```python
from build123d import *

# Parameters (mm, degrees)
SKETCH1_W           = 6.8
SKETCH1_H           = 5
BOSS_EXTRUDE1_DEPTH = 3.8
SKETCH3_W           = 2.8
SKETCH3_H           = 2.9
CUT_EXTRUDE2_DEPTH  = 10.340235543
SKETCH4_W           = 1.9
SKETCH4_H           = 0.2
CUT_EXTRUDE3_DEPTH  = 2.2
HOLE1_D             = 1.05
HOLE1_CBORE_D       = 1.3
HOLE1_CBORE_DEPTH   = 1.2
CUT_EXTRUDE8_DEPTH  = 10.340235543
CUT_EXTRUDE9_DEPTH  = 10.340235543
CUT_EXTRUDE10_DEPTH = 0.3
SKETCH20_W          = 5
SKETCH20_H          = 1.3
CUT_EXTRUDE11_DEPTH = 0.3


with BuildPart() as part:
    # Sketch1 → Boss-Extrude1 (new body)
    with BuildSketch(Plane(origin=(0, 4, 0), x_dir=(-1, 0, 0), z_dir=(0, 1, 0))):
        with Locations((-3.4, 2.5)):
            Rectangle(SKETCH1_W, SKETCH1_H)
    extrude(amount=-BOSS_EXTRUDE1_DEPTH)

    # Sketch3 → Cut-Extrude2 (cut, through all)
    with BuildSketch(Plane.XY.offset(5)):
        with Locations((3.2, 1.65)):
            Rectangle(SKETCH3_W, SKETCH3_H)
    extrude(amount=-CUT_EXTRUDE2_DEPTH, mode=Mode.SUBTRACT)

    # Sketch4 → Cut-Extrude3 (cut)
    with BuildSketch(Plane(origin=(6.8, 0, 0), x_dir=(0, 0, -1), z_dir=(1, 0, 0))):
        with Locations((-1.9, 0.3)):
            Rectangle(SKETCH4_W, SKETCH4_H)
    extrude(amount=-CUT_EXTRUDE3_DEPTH, mode=Mode.SUBTRACT)

    # Hole1 (through all)
    with Locations(Plane(origin=(0, 0, 0), x_dir=(-1, 0, 0), z_dir=(0, 0, -1))):
        with Locations((-5.7, 1.7), (-0.7, 1.7)):
            CounterBoreHole(HOLE1_D / 2, HOLE1_CBORE_D / 2, HOLE1_CBORE_DEPTH)

    # Sketch17 → Cut-Extrude8 (cut, through all)
    with BuildSketch(Plane.XY.offset(5)):
        with BuildLine():
            Line((6.8, 2.225), (5.7, 2.225))
            ThreePointArc((5.7, 2.225), (6.07123106, 2.07123106), (6.225, 1.7))
            ThreePointArc((6.225, 1.7), (6.07123106, 1.32876894), (5.7, 1.175))
            Line((5.7, 1.175), (6.8, 1.175))
            Line((6.8, 1.175), (6.8, 2.225))
        make_face()
        with BuildLine():
            ThreePointArc((6.225, 1.7), (6.07123106, 2.07123106), (5.7, 2.225))
            Line((5.7, 2.225), (5.7, 1.175))
            ThreePointArc((5.7, 1.175), (6.07123106, 1.32876894), (6.225, 1.7))
        make_face()
        with BuildLine():
            Line((5.7, 1.175), (5.7, 2.225))
            ThreePointArc((5.7, 2.225), (5.175, 1.7), (5.7, 1.175))
        make_face()
    extrude(amount=-CUT_EXTRUDE8_DEPTH, mode=Mode.SUBTRACT)

    # Sketch18 → Cut-Extrude9 (cut, through all)
    with BuildSketch(Plane(origin=(6.8, 0, 0), x_dir=(0, 0, -1), z_dir=(1, 0, 0))):
        Polygon((-1.288675135, 4), (-3.711324865, 4), (-4, 3.5), (-1, 3.5), align=None)
    extrude(amount=-CUT_EXTRUDE9_DEPTH, mode=Mode.SUBTRACT)

    # Sketch19 → Cut-Extrude10 (cut)
    with BuildSketch(Plane(origin=(0, 3.5, 0), x_dir=(1, 0, 0), z_dir=(0, 1, 0))):
        with BuildLine():
            Line((6.8, -1.75), (6, -1.75))
            ThreePointArc((6, -1.75), (6.530330086, -1.969669914), (6.75, -2.5))
            ThreePointArc((6.75, -2.5), (6.530330086, -3.030330086), (6, -3.25))
            Line((6, -3.25), (6.8, -3.25))
            Line((6.8, -3.25), (6.8, -1.75))
        make_face()
        with BuildLine():
            ThreePointArc((6.75, -2.5), (6.530330086, -1.969669914), (6, -1.75))
            Line((6, -1.75), (6, -3.25))
            ThreePointArc((6, -3.25), (6.530330086, -3.030330086), (6.75, -2.5))
        make_face()
        with BuildLine():
            Line((6, -3.25), (6, -1.75))
            ThreePointArc((6, -1.75), (5.25, -2.5), (6, -3.25))
        make_face()
    extrude(amount=-CUT_EXTRUDE10_DEPTH, mode=Mode.SUBTRACT)

    # Sketch20 → Cut-Extrude11 (cut)
    with BuildSketch(Plane(origin=(6.8, 0, 0), x_dir=(0, 0, -1), z_dir=(1, 0, 0))):
        with Locations((-2.5, 3.35)):
            Rectangle(SKETCH20_W, SKETCH20_H)
    extrude(amount=-CUT_EXTRUDE11_DEPTH, mode=Mode.SUBTRACT)


solid = part.part
```
Check sheet for the modelled part. Datum: model origin and axes. Units: mm. A direction names the side the tool comes from. Coordinates: 2 decimals unless noted, no trailing zeros. Order: outer loops, then holes, each group sorted by start corner. A loop starts at its lowest first (then second) coordinate and runs counter-clockwise, first axis right, second up. Notation, with made-up numbers: M 34.5,0.5 L 40.5,0.5 A16 cw 40.5,10.5 Z; hole C 37.25,-22 d4. An arc over 180 degrees is marked long. Write each question's results on one line, items separated by ' | '. Start each with the question number.
1. Cross-section at A-A on z = 2.5. Record the cut outline in (x, y) (3 decimals), and give its area (3 significant figures).
2. Mould release check, pull along Y, two halves, no side actions. Record for faces 1 (the face through (3, 3.5, 3)), 2 (the face through (3, 4, 1)), 3 (the face through (3.4, 3.4, 0)): +Y half, -Y half, draft (parallel to the pull), parting line (faces both ways), or undercut.
3. Access from +Z, -Z, +X, -X, +Y, -Y to the whole of each face (thin tool, end or side, straight path). Record for faces 4 (the face through (6, 0.4, 2)), 5 (the face through (6, 3.2, 2)), 6 (the face through (1.8, 2, 3)), 7 (the face through (6, 1.175, 3)).
4. Cross-section at C-C on y = 0.7. Record the cut outline in (x, z), and give its area (3 significant figures).
5. Cross-section at D-D on y = 1.7. Record the cut outline in (x, z) (3 decimals).
6. Material ranges on probe 1 along Y at (x, z) = (5.75, 0.5); probe 2 along X at (y, z) = (1.45, 4.5); probe 3 along X at (y, z) = (2.4, 4), recorded low to high.
7. Cross-section at B-B on x = 0.7. Record the cut outline in (y, z) (3 decimals), and give its area (3 significant figures).
8. Go/stop test with flat-tipped pins: P1, Ø1.5, axis at x = 0.7, y = 1.7, coming from the -Z side; P2, Ø1.5, axis at x = 6, z = 2, coming from the -Y side; P3, Ø0.9, axis at x = 6.5, z = 3, coming from the +Y side. Record where each tip stops, or that it passes through.
Checks:
1) outline: M 0,0.2 L 1.8,0.2 L 1.8,3.1 L 4.6,3.1 L 4.6,0.4 L 6.8,0.4 L 6.8,1.175 L 5.7,1.175 A0.525 cw 5.7,2.225 L 6.8,2.225 L 6.8,2.7 L 6.5,2.7 L 6.5,3.2 L 5.25,3.2 L 5.25,3.5 L 0,3.5 Z; hole C 0.7,1.7 d1.05 | area: 10.8 mm²
2) face 1: undercut | face 2: +Y half | face 3: draft
3) face 4: +X, -Y | face 5: +X, +Y | face 6: +Z, -Z, -Y | face 7: +Z, -Z, +X
4) outline: M 0,0 L 1.8,0 L 1.8,5 L 0,5 Z; M 4.6,0 L 6.8,0 L 6.8,5 L 4.6,5 Z | area: 20.0 mm²
5) outline: M 0,0 L 0.05,0 L 0.05,1.2 L 0.175,1.2 L 0.175,5 L 0,5 Z; M 1.225,1.2 L 1.35,1.2 L 1.35,0 L 1.8,0 L 1.8,5 L 1.225,5 Z; M 4.6,0 L 5.05,0 L 5.05,1.2 L 5.175,1.2 L 5.175,5 L 4.6,5 Z
6) probe 1: y = 0.2 to 1.05, 2.35 to 4 | probe 2: x = 0 to 0.24, 1.16 to 1.8, 4.6 to 5.24 | probe 3: x = 0 to 1.8, 4.6 to 6.8
7) outline: M 0.2,0 L 1.05,0 L 1.05,1.2 L 1.175,1.2 L 1.175,5 L 0.2,5 Z; M 2.225,1.2 L 2.35,1.2 L 2.35,0 L 4,0 L 4,1.289 L 3.5,1 L 3.5,4 L 4,3.711 L 4,5 L 2.225,5 Z | area: 12.1 mm²
8) P1: stops at z = 0 | P2: stops at y = 0.4 | P3: stops at y = 3.5
